Could you check a few things on this model? Use its own coordinates, in mm. A direction names the side the tool comes from. Give positions to 0.01 mm unless a question says otherwise; leave off trailing zeros. Order: outer loops, then holes, each group sorted by start corner. A loop starts at its lowest first (then second) coordinate and runs counter-clockwise, first axis right, second up. Notation, with made-up numbers: (-10, -28.5) -> (49, -28.5) arc R20 cw to (49, 7.5) -> close; hole circle Ø2 at (67.5, 45.5). An arc over 180 degrees is marked (long way). Answer as CSV lines item,"result". Start each with the question number.
(1) On a 3-axis mill with a long thin cutter (end or side, diameter ignored), from which of +Z, -Z, +X, -X, +Y, -Y can I reach the whole of each face in a straight line? I mean faces 4 (the face through (-20, -1, 47)), 5 (the face through (49, -1, -20)), 6 (the face through (-47.5, -1, -32)), 7 (the face through (20, -1, 46)). Say none if no direction works.
(2) I want a section at A-A (x = 0). Please give me the cut outline in (y, z), plus the area to 3 significant figures.
(3) I want a section at B-B (z = -9). Please give me the cut outline in (x, y).
(4) We'd pull the mould along X, two halves only. Please class faces 1 (the face through (-20, -1, -46)), 2 (the face through (-43.734, -1.479, 39.048)), 3 (the face through (0, -1, 48)): released by +X, released by -X, zero draft, split by the parting line, or undercut.
(5) I want a section at D-D (x = -43.3). Please give me the cut outline in (y, z), plus the area to 3 significant figures.
(6) I want a section at C-C (y = -0.7). Please give me the cut outline in (x, z).
(7) I need wall thicknesses on L1, parallel to Z at x = 43.3, y = -1.9; L2, parallel to Z at x = 0, y = -0.6; L3, parallel to Z at x = -4, y = -1.1. Which ranges of each line are inside material? Lowest first, please.
(8) Will these pins go through, and if not, where does the flat tip stop? pin 1 Ø1.5 at (y, z) = (-1.5, 47) entering from -X; pin 2 Ø1.5 at (y, z) = (-1, -34.5) entering from +X; pin 3 Ø1.5 at (x, y) = (49.5, -1) entering from -Z; pin 4 Ø2.5 at (x, z) = (43.3, 41) entering from +Y.
```python
from build123d import *

# Parameters (mm, degrees)
F0_R     = 2
F0_R_2   = 15
F1_DEPTH = 3


with BuildPart() as f1:
    # F0 (on Front) → F1 (new body)
    with BuildSketch(Plane.XZ):
        Polygon((-50.5, 20), (-50.5, 0), (-50.5, -20), (-47.5, -20), (-47.5, -45), (-20, -45), (-20, -48), (0, -48), (20, -48), (20, -45), (47.5, -45), (47.5, -20), (50.5, -20), (50.5, 0), (50.5, 20), (47.5, 20), (47.5, 45), (20, 45), (20, 48), (0, 48), (-20, 48), (-20, 45), (-47.5, 45), (-47.5, 20), align=None)
        with Locations((-43.3, -41)):
            Circle(F0_R, mode=Mode.SUBTRACT)
        with Locations((43.3, -41)):
            Circle(F0_R, mode=Mode.SUBTRACT)
        with Locations((-43.3, 41)):
            Circle(F0_R, mode=Mode.SUBTRACT)
        Circle(F0_R_2, mode=Mode.SUBTRACT)
        with Locations((43.3, 41)):
            Circle(F0_R, mode=Mode.SUBTRACT)
    extrude(amount=F1_DEPTH)


solid = f1.part
```
Final values:
1,face 4,"+Z, -X, +Y, -Y"
1,face 5,"-Z, +X, +Y, -Y"
1,face 6,"-Z, -X, +Y, -Y"
1,face 7,"+Z, +X, +Y, -Y"
2,outline,"(-3, -48) -> (0, -48) -> (0, -15) -> (-3, -15) -> close; (-3, 15) -> (0, 15) -> (0, 48) -> (-3, 48) -> close"
2,area,"198 mm²"
3,outline,"(-50.5, -3) -> (-12, -3) -> (-12, 0) -> (-50.5, 0) -> close; (12, -3) -> (50.5, -3) -> (50.5, 0) -> (12, 0) -> close"
4,face 1,"released by -X"
4,face 2,"undercut"
4,face 3,"zero draft"
5,outline,"(-3, -45) -> (0, -45) -> (0, -43) -> (-3, -43) -> close; (-3, -39) -> (0, -39) -> (0, 39) -> (-3, 39) -> close; (-3, 43) -> (0, 43) -> (0, 45) -> (-3, 45) -> close"
5,area,"246 mm²"
6,outline,"(-50.5, -20) -> (-47.5, -20) -> (-47.5, -45) -> (-20, -45) -> (-20, -48) -> (20, -48) -> (20, -45) -> (47.5, -45) -> (47.5, -20) -> (50.5, -20) -> (50.5, 20) -> (47.5, 20) -> (47.5, 45) -> (20, 45) -> (20, 48) -> (-20, 48) -> (-20, 45) -> (-47.5, 45) -> (-47.5, 20) -> (-50.5, 20) -> close; hole circle Ø4 at (-43.3, -41); hole circle Ø4 at (-43.3, 41); hole circle Ø30 at (0, 0); hole circle Ø4 at (43.3, -41); hole circle Ø4 at (43.3, 41)"
7,L1,"-45 to -43, -39 to 39, 43 to 45"
7,L2,"-48 to -15, 15 to 48"
7,L3,"-48 to -14.46, 14.46 to 48"
8,pin 1,"x = -20"
8,pin 2,"x = 47.5"
8,pin 3,"z = -20"
8,pin 4,"through"
